Input: part model. Units: mm. Frame: model coordinates. A direction names the side the tool comes from. Coordinates: 2 decimals unless noted, no trailing zeros. Loops run counter-clockwise (first coordinate to the right, second up) from the corner with the lowest first, then second, coordinate; pieces in that order, holes last.
Item 1: Section B-B on x = -17. Return loops of the section in (y, z), and give its area (3 significant figures).
Item 2: Section A-A on x = -2.5. Return loops of the section in (y, z).
Item 3: Contact query for flat-ended pins moving along their axis: P1, Ø2, axis at x = -22.5, y = 20, coming from the +Z side; P2, Ø10, axis at y = 23, z = 16.5, coming from the +X side; P3, Ø3, axis at x = 1, y = 6, coming from the -Z side. Output: stop coordinate, or through.
Item 4: Ray query, line 1 along Y through (x, z) = (-2.3, 0); line 2 along Y through (x, z) = (-49, -0.5); line 3 along X through (y, z) = (13, -22). Return the intervals inside material, ascending.
Item 5: Reachability of faces 1 (the flat face through (34, 0, 0)), 2 (the flat face through (21, 2, 0)), 3 (the cylindrical face through (20.818, -3.373, 2.15)) from +Z, -Z, +X, -X, +Y, -Y: full face, straight path, thin tool, end or side. Return the list, or none.
Item 6: Pull-direction query (Y, two-part tool) for faces 4 (the cylindrical face through (-40.538, 31.232, 4.101)), 5 (the cylindrical face through (-2.586, 20.364, 0.215)), 6 (the flat face through (-74, 0, 0)); classes: released by +Y, released by -Y, zero draft, split by the parting line, or undercut.
```python
from build123d import *

# Parameters (mm, degrees)
SKETCH_1_R          = 31.5
EXTRUDE_1_DEPTH     = 74
SKETCH_2_R          = 5
EXTRUDE_2_DEPTH     = 8
SKETCH_3_R          = 4
EXTRUDE_3_DEPTH     = 26
CUT_EXTRUDE_1_DEPTH = 2
M4X0_7_1_D          = 3.3
M4X0_7_1_DEPTH      = 5.1
M4X0_7_1_TIP        = 0.991420021


with BuildPart() as part:
    # 草图1 → 凸台-拉伸1 (new body)
    with BuildSketch(Plane(origin=(0, 0, 0), x_dir=(0, 0, -1), z_dir=(1, 0, 0))):
        Circle(SKETCH_1_R)
    extrude(amount=-EXTRUDE_1_DEPTH)

    # 草图2 → 凸台-拉伸2 (add)
    with BuildSketch(Plane(origin=(0, 0, 0), x_dir=(0, 0, -1), z_dir=(1, 0, 0))):
        Circle(SKETCH_2_R)
    extrude(amount=EXTRUDE_2_DEPTH)

    # 草图3 → 凸台-拉伸3 (add)
    with BuildSketch(Plane(origin=(8, 0, 0), x_dir=(0, 0, -1), z_dir=(1, 0, 0))):
        with Locations(Location((0, 0, 0), (0, 0, 180))):
            Circle(SKETCH_3_R)
    extrude(amount=EXTRUDE_3_DEPTH)

    # Sketch 3D_1 → 切除-拉伸1 (cut)
    with BuildSketch(Plane(origin=(12.5, 4, 1.5), x_dir=(0.9847835588179368, 0, -0.17378533390904766), z_dir=(0, -1, 0))):
        with BuildLine():
            Line((0, 0), (16.7413205, 2.954350676))
            ThreePointArc((16.7413205, 2.954350676), (18.479173839, 1.737853339), (17.262676502, 0))
            Line((17.262676502, 0), (0.521356002, -2.954350676))
            ThreePointArc((0.521356002, -2.954350676), (-1.216497337, -1.737853339), (0, 0))
        make_face()
    extrude(amount=CUT_EXTRUDE_1_DEPTH, mode=Mode.SUBTRACT)

    # M4x0.7 螺纹孔1
    with Locations(Plane(origin=(0, 22, 0), x_dir=(0, 0, 1), z_dir=(1, 0, 0))):
        with Locations((0, 0), (-22, 22), (0, 44), (22, 22)):
            Hole(M4X0_7_1_D / 2, depth=M4X0_7_1_DEPTH)
            with Locations((0, 0, -(M4X0_7_1_DEPTH + M4X0_7_1_TIP / 2))):  # 118° drill point
                Cone(0, M4X0_7_1_D / 2, M4X0_7_1_TIP, mode=Mode.SUBTRACT)

    # 草图9 → 切除-旋转1 (revolve, cut)
    with BuildSketch(Plane.XY, mode=Mode.PRIVATE) as cut_revolve_1_sk:
        Polygon((0, 31.5), (0, 27.5), (-8, 31.5), align=None)
    revolve(cut_revolve_1_sk.sketch.rotate(Axis((0, 0, 0), (-1, 0, 0)), 90), axis=Axis((0, 0, 0), (-1, 0, 0)), mode=Mode.SUBTRACT)


solid = part.part
```
Results found:
1. outline: circle Ø63 at (0, 0)
1. area: 3,120 mm2
2. outline: circle Ø57.5 at (0, 0); hole circle Ø3.3 at (-22, 0); hole circle Ø3.3 at (0, -22); hole circle Ø3.3 at (0, 22); hole circle Ø3.3 at (22, 0)
3. P1: stops at z = 25.12
3. P2: stops at x = 0
3. P3: stops at z = -27.16
4. line 1: y = -28.65 to -23.65, -20.35 to 20.35, 23.65 to 28.65
4. line 2: y = -31.5 to 31.5
4. line 3: x = -74 to 0
5. face 1: +Z, -Z, +X, +Y, -Y
5. face 2: +Y
5. face 3: +X
6. face 4: split by the parting line
6. face 5: undercut
6. face 6: zero draft
